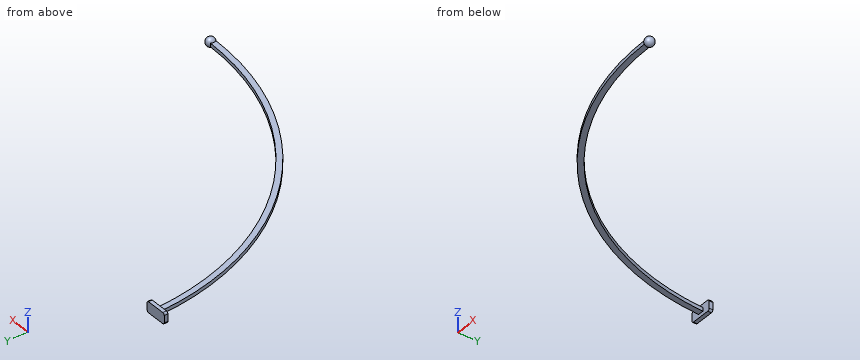
from build123d import *

# Parameters (mm, degrees)
PAD_DEPTH    = 0.25
PAD001_DEPTH = 0.5


with BuildPart() as part:
    # Sketch → Pad (new body, symmetric)
    with BuildSketch(Plane.XY):
        with BuildLine():
            Line((-0.375, 0), (0, 0))
            Line((0, 0), (0.375, 0))
            ThreePointArc((0.375, 0), (10.516428, -24.483572), (35, -34.625))
            Line((35, -34.625), (35, -35))
            Line((35, -35), (35, -35.375))
            ThreePointArc((-0.375, 0), (9.986098, -25.013902), (35, -35.375))
        make_face()
    extrude(amount=PAD_DEPTH, both=True)

    # Sketch001 (on DatumPlane) → Revolution (revolve)
    with BuildSketch(Plane(origin=(35, -35, 0), x_dir=(0, 1, 0), z_dir=(1, 0, 0))):
        with BuildLine():
            ThreePointArc((0, 0.625), (-0.625, 0), (0, -0.625))
            Line((0, 0), (0, -0.625))
            Line((0, 0.625), (0, 0))
        make_face()
    revolve(axis=Axis((35, -35, 0), (0, 0, -1)))

    # Sketch002 → Pad001 (join)
    with BuildSketch(Plane.XZ):
        with BuildLine():
            ThreePointArc((-1.25, 0.75), (-1.426777, 0.676777), (-1.5, 0.5))
            Line((-1.5, -0.5), (-1.5, 0.5))
            ThreePointArc((-1.5, -0.5), (-1.426777, -0.676777), (-1.25, -0.75))
            Line((1.25, -0.75), (-1.25, -0.75))
            ThreePointArc((1.25, -0.75), (1.426777, -0.676777), (1.5, -0.5))
            Line((1.5, 0.5), (1.5, -0.5))
            ThreePointArc((1.5, 0.5), (1.426777, 0.676777), (1.25, 0.75))
            Line((-1.25, 0.75), (1.25, 0.75))
        make_face()
    extrude(amount=PAD001_DEPTH)


solid = part.part
Could you check a few things on this model? Use its own coordinates, in mm. Give positions to 0.01 mm unless a question says otherwise; leave off trailing zeros. Order: outer loops, then holes, each group sorted by start corner. A loop starts at its lowest first (then second) coordinate and runs counter-clockwise, first axis right, second up.
Item 1: If we section it at C-C, the plane y = -21.5: Write out the boundary of the cut face in (x, z), plus the area to 3 significant figures.
Item 2: I need wall thicknesses on line 1 (Y direction, x = 7, z = -0.2); line 2 (Y direction, x = 12, z = 0.1); line 3 (X direction, y = -12, z = 0.2). Which ranges of each line are inside material? Lowest first, please.
Item 3: If we section it at A-A, the plane z = 0: Write out the boundary of the cut face in (x, y) (3 decimals).
Item 4: I'm going to push a flat-ended pin straight in: pin 1 (1.5 mm diameter, centred on x = 8, y = -19.5, fed in from +Z). Where does the tip first touch, or does it pass through?
Item 5: If we section it at B-B, the plane x = 14: Write out the boundary of the cut face in (y, z).
Values:
1. outline: (6.91, -0.25) - (7.86, -0.25) - (7.86, 0.25) - (6.91, 0.25) - close
1. area: 0.475 mm2
2. line 1: y = -21.62 to -20.37
2. line 2: y = -26.88 to -25.88
2. line 3: x = 1.72 to 2.52
3. outline: (-1.5, -0.5) - (-0.371, -0.5) arc R35.375 ccw to (34.497, -35.371) arc R0.625 ccw (long way) to (34.503, -34.621) arc R34.625 cw to (0.379, -0.5) - (1.5, -0.5) - (1.5, 0) - (-1.5, 0) - close
4. pin 1: passes through
5. outline: (-28.47, -0.25) - (-27.53, -0.25) - (-27.53, 0.25) - (-28.47, 0.25) - close
